Autodesk Inventor part; units mm, degrees
ref_plane "YZ Plane" through (0, 0, 0) normal (1, 0, 0) x (0, 1, 0)
ref_plane "XZ Plane" through (0, 0, 0) normal (0, 1, 0) x (-1, 0, 0)
ref_plane "XY Plane" through (0, 0, 0) normal (0, 0, 1) x (1, 0, 0)
sketch "Boceto1" plane through (0, 0, 0) normal (1, 0, 0) x (0, 1, 0)
  line L0 (0, 0) -> (30, 0)
  line L1 (30, 0) -> (30, -20)
  line L2 (30, -20) -> (0, -20)
  line L3 (0, -20) -> (0, 0)
  line L4 (21, -10) -> (11, -10) construction
  line L5 (21, -7) -> (11, -7)
  line L6 (11, -13) -> (21, -13)
  arc A0 (21, -13) -> (21, -7) centre (21, -10) ccw
  arc A1 (11, -7) -> (11, -13) centre (11, -10) ccw
  point P0 (16, -10)
  point P1 (24, -10)
  point P2 (30, -10)
  point P3 (0, -10)
  point P4 (8, -10)
  dimension "d0" = 30
  dimension "d1" = 20
  dimension "d2" = 10
  dimension "d3" = 6
  dimension "d4" = 6
extrude "Extrusión1" add sketch "Boceto1" along normal blind 5
sketch "Boceto2" plane through (5, 0, 0) normal (1, 0, 0) x (0, 0, -1)
  line L0 (0, 0) -> (20, 0)
  line L1 (0, 0) -> (20, 0)
  line L2 (20, 0) -> (20, 5)
  line L3 (20, 5) -> (0, 5)
  line L4 (0, 5) -> (0, 0)
  dimension "d8" = 20
  dimension "d9" = 5
extrude "Extrusión2" add sketch "Boceto2" along normal blind 25
sketch "Boceto3" plane through (5, 5, 0) normal (0, 1, 0) x (1, 0, 0)
  line L0 (6, 10) -> (16, 10) construction
  line L1 (6, 7) -> (16, 7)
  line L2 (16, 13) -> (6, 13)
  arc A0 (6, 13) -> (6, 7) centre (6, 10) ccw
  arc A1 (16, 7) -> (16, 13) centre (16, 10) ccw
  line L3 (25, 20) -> (25, 0)
  line L4 (0, 0) -> (25, 0)
  point P0 (-5, 0)
  point P1 (11, 10)
  point P2 (25, 10)
  point P3 (19, 10)
  dimension "d12" = 10
  dimension "d13" = 6
  dimension "d14" = 6
  dimension "d15" = 10
extrude "Extrusión3" cut sketch "Boceto3" against normal blind 5
sketch "Boceto4" plane through (0, 0, 0) normal (0, 0, 1) x (1, 0, 0)
  line L0 (5, 30) -> (5, 5)
  line L1 (5, 5) -> (30, 5)
  line L2 (5, 5) -> (5, 28)
  line L3 (5, 30) -> (7, 30)
  line L4 (7, 30) -> (7, 28)
  line L5 (30, 5) -> (30, 7)
  line L6 (30, 7) -> (28, 7)
  line L7 (28, 7) -> (7, 28)
  point P0 (0, 0)
  point P1 (28, 5)
  dimension "d18" = 2
  dimension "d19" = 2
  dimension "d22" = 2
extrude "Extrusión4" add sketch "Boceto4" against normal blind 2
sketch "Boceto5" plane through (0, 0, -20) normal (0, 0, -1) x (-1, 0, 0)
  line L0 (-30, 0) -> (-30, 5)
  line L1 (-30, 0) -> (-30, 7)
  line L2 (-30, 5) -> (-30, 7)
  line L3 (-30, 7) -> (-28, 7)
  line L4 (-7, 30) -> (-7, 28)
  line L5 (-28, 7) -> (-7, 28)
  line L6 (-7, 28) -> (-7, 30)
  line L7 (-7, 30) -> (-5, 30)
  line L8 (-5, 30) -> (-5, 5)
  line L9 (-5, 5) -> (-30, 5)
  point P0 (0, 0)
  dimension "d23" = 2
extrude "Extrusión5" add sketch "Boceto5" against normal blind 2
properties part number "Esquinero" material "Aluminio 6061"
Verification items for the finished model (mm, model axes). A direction names the side the tool comes from. Round coordinates to 2 decimals unless told otherwise and drop trailing zeros. Write each loop counter-clockwise with the first axis right and the second up, starting at its lowest first coordinate (ties: lowest second). Pieces come first, ordered by that corner, then holes. Notation, with made-up numbers: (-18, 57) - (16, 57) arc R37 ccw to (16, 96) - close; hole circle Ø2 at (13, 67). An arc over 180 degrees is marked (long way). Answer as a JSON object with one key per item and string values. Group by question number.
Q1. Tool access check on faces 1 (the cylindrical face through (2, 8, -10)), 2 (the flat face through (29, 7, -1)), 3 (the flat face through (5, 17.3, -13.4)), 4 (the flat face through (16, 3, -13)), 5 (the flat face through (30, 3, -10)). Record the directions out of +Z, -Z, +X, -X, +Y, -Y that give a thin tool (end or side, any length) a straight path to the whole face; none if there is none.
Q2. Go/stop test with flat-tipped pins: pin 1 Ø10 at (y, z) = (11, -8) entering from +X; pin 2 Ø1.6 at (x, z) = (28.5, -1) entering from +Y; pin 3 Ø5 at (x, z) = (19.5, -13) entering from +Y. Record where each tip stops, or that it passes through.
Q3. Section check C-C, the plane x = 11.5. Enter the section's corners in (y, z).
Q4. Section check D-D, the plane y = 2.75. Enter the section's corners in (x, z).
Q5. Thickness scan on line 1 (Z direction, x = 17, y = 13.5); line 2 (Y direction, x = 8, z = -13); line 3 (Z direction, x = 14.5, y = 4). Record the ranges inside material, lowest first.
Q6. Section check B-B, the plane y = 20.25. Enter the section's corners in (x, z).
Q7. Section check A-A, the plane z = -10. Enter the section's corners in (x, y).
Q8. Mould release check, pull along Z, two halves, no side actions. Record for faces 6 (the cylindrical face through (2, 24, -10)), 7 (the flat face through (12, 12, -20)), 8 (the flat face through (15, 0, -6)): released by +Z, released by -Z, zero draft, split by the parting line, or undercut.
Found:
{
 "1": {"face 1": "+X, -X", "face 2": "+Z, -Z, +X, +Y", "face 3": "+X, +Y", "face 4": "+Y, -Y", "face 5": "+Z, -Z, +X, +Y, -Y"},
 "2": {"pin 1": "stops at x = 5", "pin 2": "stops at y = 7.3", "pin 3": "stops at y = 5"},
 "3": {"outline": "(0, -20) - (23.5, -20) - (23.5, -18) - (5, -18) - (5, -13) - (0, -13) - close; (0, -7) - (5, -7) - (5, -2) - (23.5, -2) - (23.5, 0) - (0, 0) - close"},
 "4": {"outline": "(0, -20) - (30, -20) - (30, 0) - (0, 0) - close; hole (11, -13) - (21, -13) arc R3 ccw to (21, -7) - (11, -7) arc R3 ccw to start"},
 "5": {"line 1": "z = -20 to -18, -2 to 0", "line 2": "y = 0 to 5", "line 3": "z = -20 to -13, -7 to 0"},
 "6": {"outline": "(0, -20) - (14.75, -20) - (14.75, -18) - (5, -18) - (5, -13) - (0, -13) - close; (0, -7) - (5, -7) - (5, -2) - (14.75, -2) - (14.75, 0) - (0, 0) - close"},
 "7": {"outline": "(0, 0) - (8, 0) - (8, 5) - (5, 5) - (5, 8) - (0, 8) - close; (0, 24) - (5, 24) - (5, 30) - (0, 30) - close; (24, 0) - (30, 0) - (30, 5) - (24, 5) - close"},
 "8": {"face 6": "undercut", "face 7": "released by -Z", "face 8": "zero draft"}
}
